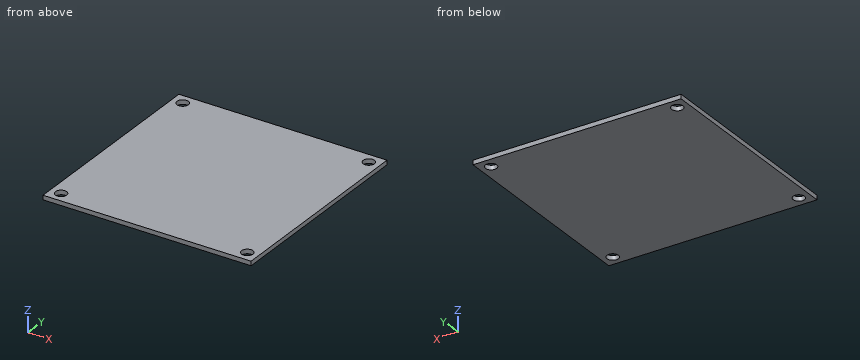
Autodesk Fusion 360 part; units mm, degrees
sketch "Module Outline" plane through (0, 0, 0) normal (0, 0, 1) x (1, 0, 0)
  line L0 (-120.65, -120.65) -> (120.65, -120.65)
  line L1 (120.65, -120.65) -> (120.65, 120.65)
  line L2 (120.65, 120.65) -> (-120.65, 120.65)
  line L3 (-120.65, 120.65) -> (-120.65, -120.65)
  line L4 (-120.65, -120.65) -> (120.65, 120.65) construction
  line L5 (120.65, -120.65) -> (-120.65, 120.65) construction
  dimension "d17" = 241.3
  dimension "d18" = 241.3
extrude "Shelf Plate" add sketch "Module Outline" along normal blind 5.08
sketch "Anchor Locations" plane through (0, 0, 5.08) normal (0, 0, 1) x (1, 0, 0)
  line L0 (-120.65, 120.65) -> (-120.65, -120.65)
  line L1 (-120.65, -120.65) -> (120.65, -120.65)
  line L2 (120.65, -120.65) -> (120.65, 120.65)
  line L3 (120.65, 120.65) -> (-120.65, 120.65)
  line L4 (120.65, 120.65) -> (107.95, 107.95) construction
  line L5 (120.65, -120.65) -> (120.65, 120.65) construction
  line L6 (-120.65, -120.65) -> (120.65, -120.65) construction
  line L7 (-120.65, 120.65) -> (-120.65, -120.65) construction
  line L8 (120.65, 120.65) -> (-120.65, 120.65) construction
  line L9 (0, 134.6139) -> (0, -139.7)
  point P0 (-107.95, 107.95)
  dimension "d22" = 12.7
  dimension "d23" = 12.7
sketch "Socket Geometry" plane through (0, 0, 5.08) normal (0, 0, 1) x (1, 0, 0)
  line L0 (-120.65, 120.65) -> (-120.65, -120.65)
  line L1 (-120.65, -120.65) -> (120.65, -120.65)
  line L2 (120.65, -120.65) -> (120.65, 120.65)
  line L3 (120.65, 120.65) -> (-120.65, 120.65)
  circle A0 centre (107.95, 107.95) radius 6.5532
  line L4 (0, 127) -> (0, -127)
  circle A1 centre (-107.95, 107.95) radius 6.5532
  line L5 (-130.6691, 0) -> (143.6907, 0)
  circle A2 centre (107.95, -107.95) radius 6.5532
  circle A3 centre (-107.95, -107.95) radius 6.5532
  point P0 (107.95, 107.95)
  point P1 (-101.6, 101.6)
  point P2 (-101.6, -101.6)
  point P3 (101.6, -101.6)
  dimension "d28" = 13.1064
extrude "Socket Cut" cut sketch "Socket Geometry" against normal blind 7.62 contours A0 | A1 | A2 | A3
equation "shelfLength = 12 in"
equation "shelfDepth = 8 in"
equation "shelfThickness = 0.20 in"
equation "lipHeight = 1 in"
equation "cornerRadius = 0.5 in"
equation "clearance = 0.008 in"
equation "tileWidth = 9.5 in"
equation "tileDepth = 9.5 in"
equation "tileThickness = 0.2 in"
equation "columnSocketDiameter = 0.75 in"
equation "columnDiameter = 0.7 in"
equation "socketInset = 0.5 in"
equation "socketDepth = 0.3 in"
equation "socketWall = 0.12 in"
equation "filletSmall = 0.06 in"
equation "filletMedium = 0.12 in"
equation "d17 = tileWidth"
equation "d18 = tileDepth"
equation "d19 = shelfThickness"
equation "anchorOffset = 0.5 in"
equation "d22 = anchorOffset"
equation "d23 = anchorOffset"
equation "pinDiameter = 0.5 in"
equation "socketDiameter = pinDiameter + ( 2 * clearance )"
equation "d28 = socketDiameter"
The listing builds one solid part. Answer for the finished solid, in the listing's coordinates (mm). Coordinates: 2 decimals unless noted, no trailing zeros. Order: outer loops, then holes, each group sorted by start corner. A loop starts at its lowest first (then second) coordinate and runs counter-clockwise, first axis right, second up. Notation, with made-up numbers: M -7,-35 L 44,-35 A35 ccw 44,3 Z; hole C -0.5,-13.5 d1. An arc over 180 degrees is marked long. Answer as a JSON object with one key per item and string values. Group by question number.
1. Section A-A on x = -107.95 is taken. Write down the section's boundary in (y, z).
2. Flat-ended cylindrical pins translate along their axes: P1, Ø21, axis at x = 107.95, y = -107.95, coming from the -Z side; P2, Ø10.5, axis at x = -107.95, y = -107.95, coming from the -Z side. Find the tip coordinate at first contact, or state that the pin passes through.
3. A straight line is drawn through the part: line 1 (Y direction, x = 107.95, z = 2.55). Find the intervals that lie inside material, in ascending order.
Values follow:
{
 "1": {"outline": "M -120.65,0 L -114.5,0 L -114.5,5.08 L -120.65,5.08 Z; M -101.4,0 L 101.4,0 L 101.4,5.08 L -101.4,5.08 Z; M 114.5,0 L 120.65,0 L 120.65,5.08 L 114.5,5.08 Z"},
 "2": {"P1": "z = 0", "P2": "through"},
 "3": {"line 1": "-120.65 to -114.5, -101.4 to 101.4, 114.5 to 120.65"}
}
